Work out the finished part from the listing and answer in its coordinate system (mm). A direction names the side the tool comes from. Give positions to 0.01 mm unless a question says otherwise; leave off trailing zeros. Order: outer loops, then holes, each group sorted by start corner. A loop starts at its lowest first (then second) coordinate and runs counter-clockwise, first axis right, second up. Notation, with made-up numbers: (58.25, 61.25) - (83.25, 61.25) arc R25 ccw to (83.25, 81.25) - close; hole circle Ø10 at (38, -13). An arc over 180 degrees is marked (long way). Put each result on its own line as item: value.
Autodesk Inventor part; units mm, degrees
ref_plane "YZ Plane" through (0, 0, 0) normal (1, 0, 0) x (0, 1, 0)
ref_plane "XZ Plane" through (0, 0, 0) normal (0, 1, 0) x (-1, 0, 0)
ref_plane "XY Plane" through (0, 0, 0) normal (0, 0, 1) x (1, 0, 0)
sketch "Sketch1" plane through (0, 0, 0) normal (0, 1, 0) x (-1, 0, 0)
  line L0 (0, 0) -> (0, -65) construction
  line L1 (-5, -5) -> (-5, -60) construction
  line L2 (5, -60) -> (5, -5) construction
  arc A0 (5, -5) -> (-5, -5) centre (0, -5) ccw construction
  arc A1 (-5, -60) -> (5, -60) centre (0, -60) ccw construction
  line L3 (5.2, -60) -> (5.2, -5)
  arc A2 (5.2, -5) -> (-5.2, -5) centre (0, -5) ccw
  line L4 (-5.2, -5) -> (-5.2, -60)
  arc A3 (-5.2, -60) -> (5.2, -60) centre (0, -60) ccw
  arc A4 (7.2, 3) -> (-7.2, 3) centre (0, 3) ccw
  line L5 (-7.2, 3) -> (-7.2, -68)
  arc A5 (-7.2, -68) -> (7.2, -68) centre (0, -68) ccw
  line L6 (7.2, -68) -> (7.2, 3)
  circle A6 centre (0, -70.2) radius 1.5
  line L7 (0, -75.2) -> (0, -65.2) construction
  circle A7 centre (0, 5.2) radius 1.5
  line L8 (0, 0.2) -> (0, 10.2) construction
  circle A8 centre (0, 5.2) radius 3
  arc A9 (-7.2, -5) -> (-5.2, -5) centre (-6.2, -5) ccw
  arc A10 (5.2, -5) -> (7.2, -5) centre (6.2, -5) ccw
  point P0 (0, -32.5)
  point P1 (7.2, -32.5)
  point P2 (0, -70.2)
  dimension "d0" = 65
  dimension "d1" = 10
  dimension "d2" = 0.2
  dimension "d8" = 2
  dimension "d9" = 2
  dimension "d10" = 10
  dimension "d11" = 10
  dimension "d12" = 3
  dimension "d13" = 3
  dimension "d14" = 6
extrude "Extrusion3" add sketch "Sketch1" along normal blind 1 contours A3 L4 A2 L3 | L3 A10 L6 A5 L5 A9 L4 A3 | A2 A9 L5 A4 L6 A10 | A8
extrude "Extrusion4" add sketch "Sketch1" along normal blind 2 from surface at 1 contours L3 A10 L6 A5 L5 A9 L4 A3 | A2 A9 L5 A4 L6 A10
extrude "Extrusion5" add sketch "Sketch1" along normal blind 2 from surface at 3 contours A2 A9 L5 A4 L6 A10
properties part number "magnet_holder"
(1) Section A-A, the plane y = 3.9 is taken. Write down the section's boundary in (x, z), then the cut area to 3 significant figures.
Geometry check:
outline: (-7.2, -5) arc R1 ccw to (-5.2, -5) arc R5.2 cw to (5.2, -5) arc R1 ccw to (7.2, -5) - (7.2, 3) arc R7.2 ccw to (-7.2, 3) - close; hole circle Ø6 at (0, 5.2)
area: 129 mm²
(2) A tool of negligible diameter and unlimited length cuts with its end or side. For faces 1 (the face through (-1, 1, 7)), 2 (the face through (-6.2, 4, -6)), 3 (the face through (0.195, 0.493, 3.713)), from which of +Z, -Z, +X, -X, +Y, -Y can it reach the whole face along a straight path? Write none if from no direction.
Geometry check:
face 1: +Y
face 2: -Z, +Y
face 3: +Y, -Y
(3) Determine the mould class of faces 4 (the face through (6.2, 4, -6)), 5 (the face through (5.4, 3, -45.1)), 6 (the face through (7.2, 1, -32)) for opening direction X: pulls with the +X half, pulls with the -X half, needs draft (parallel to the pull), parting line crosses it, or undercut.
Geometry check:
face 4: undercut
face 5: needs draft
face 6: pulls with the +X half
(4) Section B-B, the plane z = -3 is taken. Write down the section's boundary in (x, y).
Geometry check:
outline: (-7.2, 0) - (7.2, 0) - (7.2, 5) - (4.8, 5) - (4.8, 1) - (-4.8, 1) - (-4.8, 5) - (-7.2, 5) - close
(5) Straight lines are drawn through the part: line 1 (Z direction, x = 0, y = 0.5); line 2 (Z direction, x = 0, y = 1.25); line 3 (Z direction, x = 0, y = 3.2). For each, find the intervals that lie inside material, in ascending order.
Geometry check:
line 1: z = -75.2 to -71.7, -68.7 to 3.7, 6.7 to 10.2
line 2: z = -75.2 to -71.7, -68.7 to -65.2, 0.2 to 2.2, 8.2 to 10.2
line 3: z = 0.2 to 2.2, 8.2 to 10.2
(6) Section C-C, the plane x = -6.2 is taken. Write down the section's boundary in (y, z).
Geometry check:
outline: (0, -71.66) - (3, -71.66) - (3, -6) - (5, -6) - (5, 6.66) - (0, 6.66) - close
(7) Given pin 1 (1.8 mm diameter, centred on x = 1, z = 4, fed in from +Y); pin 2 (2.5 mm diameter, centred on x = 0, z = 5.2, fed in from -Y), each flat-ended and moving along its own axis, determine where each tip first touches the part or whether it passes through.
Geometry check:
pin 1: stops at y = 1
pin 2: passes through
